Source: CAD feature listing. Evaluate the final solid. Frame: model axes, mm. Give positions to 0.01 mm unless a question says otherwise; leave off trailing zeros. Loops run counter-clockwise (first coordinate to the right, second up) from the corner with the lowest first, then second, coordinate; pieces in that order, holes last. Notation, with made-up numbers: (52, 71.25) -> (74, 71.25) arc R13 cw to (74, 92.25) -> close; hole circle Ø6 at (15.25, 49). An arc over 180 degrees is marked (long way). Put each result on its own line as item: value.
```python
from build123d import *

# Parameters (mm, degrees)
F0_W     = 76.2
F0_H     = 139.7
F0_R     = 1.9812
F0_R_2   = 4.7625
F1_DEPTH = 3.175
F2_R     = 3.175
F3_DEPTH = 3.176


with BuildPart() as f1:
    # F0 (on Front) → F1 (new body)
    with BuildSketch(Plane.XZ):
        with Locations((0, -44.45)):
            Rectangle(F0_W, F0_H)
        with Locations((-26.035, 0)):
            Circle(F0_R, mode=Mode.SUBTRACT)
        Circle(F0_R_2, mode=Mode.SUBTRACT)
        with Locations((26.035, 0)):
            Circle(F0_R, mode=Mode.SUBTRACT)
    extrude(amount=F1_DEPTH)

    # F2 (on face) → F3 (cut, through all)
    with BuildSketch(Plane.XZ.offset(3.175)):
        with Locations((19.05, -85.725)):
            Circle(F2_R)
        with Locations((19.05, -104.775)):
            Circle(F2_R)
        with Locations((-19.05, -85.725)):
            Circle(F2_R)
        with Locations((-19.05, -104.775)):
            Circle(F2_R)
    extrude(amount=-F3_DEPTH, mode=Mode.SUBTRACT)


solid = f1.part
```
(1) Section B-B on z = 0. Return loops of the section in (x, y) (1 decimal).
Calculated:
outline: (-38.1, -3.2) -> (-28, -3.2) -> (-28, 0) -> (-38.1, 0) -> close; (-24.1, -3.2) -> (-4.8, -3.2) -> (-4.8, 0) -> (-24.1, 0) -> close; (4.8, -3.2) -> (24.1, -3.2) -> (24.1, 0) -> (4.8, 0) -> close; (28, -3.2) -> (38.1, -3.2) -> (38.1, 0) -> (28, 0) -> close
(2) Line query: probe 1 along Z at (x, y) = (19.05, -1.9); probe 2 along Z at (x, y) = (0, -1.2); probe 3 along Z at (x, y) = (-21, -1.75). Output: solid intervals per line, ascending. Write a range as from..to.
Calculated:
probe 1: z = -114.3..-107.95, -101.6..-88.9, -82.55..25.4
probe 2: z = -114.3..-4.76, 4.76..25.4
probe 3: z = -114.3..-107.28, -102.27..-88.23, -83.22..25.4
(3) First-contact query: P1, Ø8, axis at x = 24.5, z = -34.5, coming from the +Y side; P2, Ø4, axis at x = 19.05, z = -85.725, coming from the +Y side. Flat tips, straight axial feed; report the tip coordinate or a pass-through.
Calculated:
P1: stops at y = 0
P2: passes through
(4) Section C-C on x = 0. Return loops of the section in (y, z) (1 decimal), then the cut area to 3 significant figures.
Calculated:
outline: (-3.2, -114.3) -> (0, -114.3) -> (0, -4.8) -> (-3.2, -4.8) -> close; (-3.2, 4.8) -> (0, 4.8) -> (0, 25.4) -> (-3.2, 25.4) -> close
area: 413 mm²
(5) Section A-A on x = -19.05. Return loops of the section in (y, z) (3 decimals).
Calculated:
outline: (-3.175, -114.3) -> (0, -114.3) -> (0, -107.95) -> (-3.175, -107.95) -> close; (-3.175, -101.6) -> (0, -101.6) -> (0, -88.9) -> (-3.175, -88.9) -> close; (-3.175, -82.55) -> (0, -82.55) -> (0, 25.4) -> (-3.175, 25.4) -> close
(6) Draft query along Z for faces 1 (the cylindrical face through (-19.738, -1.61, -107.874)), 2 (the flat face through (-1, 0, -43)), 3 (the flat face through (-1, -2, -114.3)). Return one class per face: released by +Z, released by -Z, zero draft, split by the parting line, or undercut.
Calculated:
face 1: undercut
face 2: zero draft
face 3: released by -Z
(7) Section D-D on y = -0.9. Give the number of separate pieces and of enclosed holes in the cut face, then the cut area to 3 significant figures.
Calculated:
separate pieces: 1
enclosed holes: 7
area: 10,400 mm²
